Autodesk Fusion 360 part; units mm, degrees
sketch "スケッチ1" plane through (0, 0, 0) normal (0, 0, 1) x (1, 0, 0)
  line L0 (6.5, 127.8402) -> (6.5, 22.1598)
  line L1 (0, 150) -> (0, 0)
  line L2 (0, 0) -> (75, 0)
  line L3 (15.6284, 12.1979) -> (75, 7.0035)
  arc A0 (6.5, 22.1598) -> (15.6284, 12.1979) centre (16.5, 22.1598) ccw
  line L4 (75, 7.0035) -> (75, 0)
  line L5 (75, 142.9965) -> (15.6284, 137.8021)
  line L6 (0, 150) -> (75, 150)
  arc A1 (15.6284, 137.8021) -> (6.5, 127.8402) centre (16.5, 127.8402) ccw
  line L7 (75, 150) -> (75, 142.9965)
extrude "押し出し1" add sketch "スケッチ1" along normal blind 100
Can you work these out from the model? Positions are in its coordinate system, mm. A direction names the side the tool comes from. Give positions to 0.01 mm unless a question says otherwise; leave off trailing zeros. Loops run counter-clockwise (first coordinate to the right, second up) from the corner with the lowest first, then second, coordinate; pieces in that order, holes last. Notation, with made-up numbers: (-23, -38.75) -> (16, -38.75) arc R28 ccw to (16, -8.75) -> close; hole circle Ø10 at (78, -16). An arc over 180 degrees is marked (long way). Return JSON: item names as keys, results as strings.
Q1. I want a section at A-A, the plane x = 43. List the corners of the cut face in (y, z) for me, then the cut area to 3 significant figures.
Checks:
{"outline": "(0, 0) -> (9.8, 0) -> (9.8, 100) -> (0, 100) -> close; (140.2, 0) -> (150, 0) -> (150, 100) -> (140.2, 100) -> close", "area": "1,960 mm2"}
Q2. I need wall thicknesses on probe 1 along X at (y, z) = (44, 80); probe 2 along Y at (x, z) = (54.5, 63); probe 3 along Y at (x, z) = (40.5, 5.5). Which ranges of each line are inside material? Lowest first, please.
Checks:
{"probe 1": "x = 0 to 6.5", "probe 2": "y = 0 to 8.8, 141.2 to 150", "probe 3": "y = 0 to 10.02, 139.98 to 150"}
Q3. On a 3-axis mill with a long thin cutter (end or side, diameter ignored), from which of +Z, -Z, +X, -X, +Y, -Y can I reach the whole of each face in a straight line? I mean faces 4 (the face through (4, 81, 100)), 5 (the face through (9.198, 15.328, 49.3)). Say none if no direction works.
Checks:
{"face 4": "+Z, +X, -X, +Y, -Y", "face 5": "+Z, -Z, +X"}
Q4. We'd pull the mould along Y, two halves only. Please class faces 1 (the face through (75, 4, 49)), 2 (the face through (37, 150, 49)), 3 (the face through (45.73, 140.436, 49.3)): released by +Y, released by -Y, zero draft, split by the parting line, or undercut.
Checks:
{"face 1": "zero draft", "face 2": "released by +Y", "face 3": "undercut"}
Q5. I want a section at B-B, the plane z = 20. List the corners of the cut face in (x, y) for me.
Checks:
{"outline": "(0, 0) -> (75, 0) -> (75, 7) -> (15.63, 12.2) arc R10 cw to (6.5, 22.16) -> (6.5, 127.84) arc R10 cw to (15.63, 137.8) -> (75, 143) -> (75, 150) -> (0, 150) -> close"}
Q6. I want a section at D-D, the plane x = 60.5. List the corners of the cut face in (y, z) for me.
Checks:
{"outline": "(0, 0) -> (8.27, 0) -> (8.27, 100) -> (0, 100) -> close; (141.73, 0) -> (150, 0) -> (150, 100) -> (141.73, 100) -> close"}
Q7. For pin 1 Ø1.5 at (y, z) = (104, 50.5) entering from +X; pin 2 Ø5 at (y, z) = (105.5, 84) entering from -X, each with a flat end and sliding along its axis, tell me the tip position at first contact or that it passes through.
Checks:
{"pin 1": "stops at x = 6.5", "pin 2": "stops at x = 0"}
Q8. I want a section at C-C, the plane y = 38.5. List the corners of the cut face in (x, z) for me, then the cut area to 3 significant figures.
Checks:
{"outline": "(0, 0) -> (6.5, 0) -> (6.5, 100) -> (0, 100) -> close", "area": "650 mm2"}
